Geometry check sheet. Reference: the model listing, model coordinates, mm. A direction names the side the tool comes from. Round coordinates to 2 decimals unless told otherwise and drop trailing zeros. Order: outer loops, then holes, each group sorted by start corner. A loop starts at its lowest first (then second) coordinate and runs counter-clockwise, first axis right, second up. Notation, with made-up numbers: (30.25, 68.5) - (78.25, 68.5) arc R16 cw to (78.25, 78.5) - close; hole circle Ø6 at (21, -35). An arc over 180 degrees is marked (long way). Use a Markdown table: item, result. Add a question column.
(1) Thickness scan on line 1 along Y through (x, z) = (2, 6.25); line 2 along X through (y, z) = (-14, 8). Record the ranges inside material, lowest first. Write a range as [from, to].
(2) Section check B-B on y = 7.5. Record the boundary of the cut face in (x, z), then the cut area to 3 significant figures.
(3) Section check A-A on z = 7. Record the boundary of the cut face in (x, y).
(4) Access from +Z, -Z, +X, -X, +Y, -Y to the whole of each face (thin tool, end or side, straight path). Record for faces 1 (the face through (14.75, 0, 6)), 2 (the face through (11.72, 11.65, 7.78)), 3 (the face through (0, -14.75, 6)).
(5) Gauge pin test, flat ends, axial feed: P1, Ø17, axis at x = -3, y = -0.5, coming from the +Z side; P2, Ø5, axis at x = 2.5, z = 7, coming from the +Y side; P3, Ø1.7, axis at y = 5.5, z = 4.5, coming from the -X side. Record the tip position at first contact, or that the pin passes through.
(6) Mould release check, pull along Y, two halves, no side actions. Record for faces 4 (the face through (0, 14.75, 6)), 5 (the face through (0, 0, 3)), 6 (the face through (16, 0, 1)): released by +Y, released by -Y, zero draft, split by the parting line, or undercut.
```python
from build123d import *

# Parameters (mm, degrees)
F0_W     = 32
F0_H     = 32
F0_W_2   = 29.5
F0_H_2   = 29.5
F0_W_3   = 26.3
F0_H_3   = 26.3
F1_DEPTH = 3
F2_DEPTH = 10
F3_R     = 5
F4_SIZE  = 1.2
F5_R     = 2.5


with BuildPart() as f1:
    # F0 (on Top) → F1 (new body)
    with BuildSketch(Plane.XY):
        Rectangle(F0_W, F0_H)
        Rectangle(F0_W_2, F0_H_2, mode=Mode.SUBTRACT)
        Rectangle(F0_W_2, F0_H_2)
        Rectangle(F0_W_3, F0_H_3, mode=Mode.SUBTRACT)
        Rectangle(F0_W_3, F0_H_3)
    extrude(amount=F1_DEPTH)

    # F0 (on Top) → F2 (join)
    with BuildSketch(Plane.XY):
        Rectangle(F0_W_2, F0_H_2)
        Rectangle(F0_W_3, F0_H_3, mode=Mode.SUBTRACT)
    extrude(amount=F2_DEPTH)

    # F3
    f3_edges = [f1.edges().sort_by_distance(p)[0] for p in [
        (-13.15, 13.15, 6.5),
        (13.15, 13.15, 6.5),
        (13.15, -13.15, 6.5),
        (-13.15, -13.15, 6.5),
    ]]
    fillet(f3_edges, radius=F3_R)

    # F4
    f4_edges = [f1.edges().sort_by_distance(p)[0] for p in [
        (-14.75, 0, 10),
        (0, -14.75, 10),
        (0, 14.75, 10),
        (14.75, 0, 10),
    ]]
    chamfer(f4_edges, length=F4_SIZE)

    # F5
    f5_edges = [f1.edges().sort_by_distance(p)[0] for p in [
        (11.685534, 11.685534, 3),
    ]]
    fillet(f5_edges, radius=F5_R)


solid = f1.part
```
Check sheet entries:
| question | item | result |
|---|---|---|
| 1 | line 1 | y = [-14.75, -13.15], [13.15, 14.75] |
| 1 | line 2 | x = [-14.75, 14.75] |
| 2 | outline | (-16, 0) - (16, 0) - (16, 3) - (14.75, 3) - (14.75, 8.8) - (13.55, 10) - (13.15, 10) - (13.15, 5.5) arc R2.5 cw to (10.65, 3) - (-10.65, 3) arc R2.5 cw to (-13.15, 5.5) - (-13.15, 10) - (-13.55, 10) - (-14.75, 8.8) - (-14.75, 3) - (-16, 3) - close |
| 2 | area | 120 mm2 |
| 3 | outline | (-14.75, -14.75) - (14.75, -14.75) - (14.75, 14.75) - (-14.75, 14.75) - close; hole (-13.15, -8.15) arc R5 ccw to (-8.15, -13.15) - (8.15, -13.15) arc R5 ccw to (13.15, -8.15) - (13.15, 8.15) arc R5 ccw to (8.15, 13.15) - (-8.15, 13.15) arc R5 ccw to (-13.15, 8.15) - close |
| 4 | face 1 | +Z, +X, +Y, -Y |
| 4 | face 2 | +Z |
| 4 | face 3 | +Z, +X, -X, -Y |
| 5 | P1 | stops at z = 3.15 |
| 5 | P2 | stops at y = 14.75 |
| 5 | P3 | stops at x = -14.75 |
| 6 | face 4 | released by +Y |
| 6 | face 5 | undercut |
| 6 | face 6 | zero draft |
